Design review of the part built by this model. Coordinates are the model's own, in mm. Give positions to 0.01 mm unless a question says otherwise; leave off trailing zeros. Loops run counter-clockwise (first coordinate to the right, second up) from the corner with the lowest first, then second, coordinate; pieces in that order, holes last. Notation, with made-up numbers: (88.25, -21.75) - (144.25, -21.75) arc R27 cw to (144.25, 10.25) - close; hole circle Ø7 at (27.25, -19). An arc over 180 degrees is marked (long way). Write each question's results on one line, items separated by ' | '.
from build123d import *

# Parameters (mm, degrees)
SKETCH1_W           = 10.16
SKETCH1_H           = 5
SKETCH1_W_2         = 0.65
SKETCH1_H_2         = 0.65
BOSS_EXTRUDE1_DEPTH = 2.54
SKETCH2_W           = 0.65
SKETCH2_H           = 0.65
BOSS_EXTRUDE2_DEPTH = 9


with BuildPart() as part:
    # Sketch1 → Boss-Extrude1 (new body)
    with BuildSketch(Plane(origin=(0, 0, 0), x_dir=(1, 0, 0), z_dir=(0, 1, 0))):
        with Locations((5.08, 2.5)):
            Rectangle(SKETCH1_W, SKETCH1_H)
        with Locations((1.27, 3.77)):
            Rectangle(SKETCH1_W_2, SKETCH1_H_2, mode=Mode.SUBTRACT)
        with Locations((1.27, 1.23)):
            Rectangle(SKETCH1_W_2, SKETCH1_H_2, mode=Mode.SUBTRACT)
        with Locations((3.81, 3.77)):
            Rectangle(SKETCH1_W_2, SKETCH1_H_2, mode=Mode.SUBTRACT)
        with Locations((6.35, 3.77)):
            Rectangle(SKETCH1_W_2, SKETCH1_H_2, mode=Mode.SUBTRACT)
        with Locations((8.89, 3.77)):
            Rectangle(SKETCH1_W_2, SKETCH1_H_2, mode=Mode.SUBTRACT)
        with Locations((3.81, 1.23)):
            Rectangle(SKETCH1_W_2, SKETCH1_H_2, mode=Mode.SUBTRACT)
        with Locations((6.35, 1.23)):
            Rectangle(SKETCH1_W_2, SKETCH1_H_2, mode=Mode.SUBTRACT)
        with Locations((8.89, 1.23)):
            Rectangle(SKETCH1_W_2, SKETCH1_H_2, mode=Mode.SUBTRACT)
    extrude(amount=BOSS_EXTRUDE1_DEPTH)

    # Sketch2 → Boss-Extrude2 (add)
    with BuildSketch(Plane(origin=(0, -3, 0), x_dir=(-1, 0, 0), z_dir=(0, -1, 0))):
        with Locations((-8.89, 3.77)):
            Rectangle(SKETCH2_W, SKETCH2_H)
        with Locations((-6.35, 1.23)):
            Rectangle(SKETCH2_W, SKETCH2_H)
        with Locations((-6.35, 3.77)):
            Rectangle(SKETCH2_W, SKETCH2_H)
        with Locations((-3.81, 1.23)):
            Rectangle(SKETCH2_W, SKETCH2_H)
        with Locations((-3.81, 3.77)):
            Rectangle(SKETCH2_W, SKETCH2_H)
        with Locations((-1.27, 1.23)):
            Rectangle(SKETCH2_W, SKETCH2_H)
        with Locations((-8.89, 1.23)):
            Rectangle(SKETCH2_W, SKETCH2_H)
        with Locations((-1.27, 3.77)):
            Rectangle(SKETCH2_W, SKETCH2_H)
    extrude(amount=-BOSS_EXTRUDE2_DEPTH)


solid = part.part
(1) Insertion check: P1, Ø0.5, axis at y = -1, z = -1.5, coming from the -X side (3 decimals); P2, Ø0.7, axis at x = 6.5, y = -2, coming from the +Z side (3 decimals); P3, Ø0.7, axis at x = 1.5, y = -1.5, coming from the -Z side (3 decimals). Each pin has a flat end and moves straight along its axis. Give the tip position at first contact, or say it passes through.
Answers below:
P1: x = 0.945 | P2: z = -0.905 | P3: z = -4.095
(2) Draft analysis for pull direction X (two halves, no side actions). For faces 1 (the flat face through (0, 1, -2)), 2 (the flat face through (5, 1, -5)), 3 (the flat face through (10.16, 1, -2)), 4 (the flat face through (5, 0, -3)), state which applies: pulls with the +X half, pulls with the -X half, needs draft (parallel to the pull), parting line crosses it, or undercut.
Answers below:
face 1: pulls with the -X half | face 2: needs draft | face 3: pulls with the +X half | face 4: undercut
(3) Wall thickness on line 1 along X through (y, z) = (4.25, -3.8) (3 decimals); line 2 along Y through (x, z) = (3.5, -4.2): over which ranges is each line inside the solid? List them lowest first. Write a range as from..to.
Answers below:
line 1: 0.945..1.595, 3.485..4.135, 6.025..6.675, 8.565..9.215 | line 2: 0..2.54
(4) Take a section at B-B on x = 8.75. Give the boundary of the cut face in (y, z) (3 decimals).
Answers below:
outline: (-3, -4.095) - (0, -4.095) - (0, -5) - (2.54, -5) - (2.54, -4.095) - (6, -4.095) - (6, -3.445) - (2.54, -3.445) - (2.54, -1.555) - (6, -1.555) - (6, -0.905) - (2.54, -0.905) - (2.54, 0) - (0, 0) - (0, -0.905) - (-3, -0.905) - (-3, -1.555) - (0, -1.555) - (0, -3.445) - (-3, -3.445) - close
(5) Take a section at C-C on z = -1.75. Give the boundary of the cut face in (x, y), plus the area to 3 significant figures.
Answers below:
outline: (0, 0) - (10.16, 0) - (10.16, 2.54) - (0, 2.54) - close | area: 25.8 mm2
(6) Take a section at A-A on y = -1.75. Count the separate pieces of the cut face and the enclosed holes in it, plus the area to 3 significant figures.
Answers below:
separate pieces: 8 | enclosed holes: 0 | area: 3.38 mm2
(7) Take a section at D-D on x = 2.75. Give the boundary of the cut face in (y, z).
Answers below:
outline: (0, -5) - (2.54, -5) - (2.54, 0) - (0, 0) - close
